```python
from build123d import *

# Parameters (mm, degrees)
CROQUIS2_R              = 10
SALIENTE_EXTRUIR1_DEPTH = 30
SALIENTE_EXTRUIR2_DEPTH = 2.5
CROQUIS4_W              = 3.81
CROQUIS4_H              = 5
CROQUIS5_W              = 70
CROQUIS5_H              = 20
SALIENTE_EXTRUIR3_DEPTH = 10
CORTAR_EXTRUIR1_DEPTH   = 20


with BuildPart() as part:
    # Croquis2 → Saliente-Extruir1 (new, symmetric)
    with BuildSketch(Plane(origin=(0, 0, 0), x_dir=(1, 0, 0), z_dir=(0, 1, 0))):
        with Locations(Location((0, 0, 0), (0, 0, 270))):
            Circle(CROQUIS2_R)
    extrude(amount=SALIENTE_EXTRUIR1_DEPTH, both=True)

    # Croquis3 → Saliente-Extruir2 (add, symmetric)
    with BuildSketch(Plane.XY):
        with BuildLine():
            Line((-1.082739864, -40.663757777), (-7.62, -30))
            Line((-7.62, -30), (7.62, -30))
            Line((7.62, -30), (1.082739864, -40.663757777))
            ThreePointArc((1.082739864, -40.663757777), (0, -41.27), (-1.082739864, -40.663757777))
        make_face()
    extrude(amount=SALIENTE_EXTRUIR2_DEPTH, both=True)

    # Croquis4 → Revoluci_n1 (revolve)
    with BuildSketch(Plane.XY, mode=Mode.PRIVATE) as revoluci_n1_sk:
        with Locations((11.905, -22.5)):
            Rectangle(CROQUIS4_W, CROQUIS4_H)
    revolve(revoluci_n1_sk.sketch.rotate(Axis((0, -30, 0), (0, -1, 0)), 90), axis=Axis((0, -30, 0), (0, -1, 0)))

    # Croquis5 → Saliente-Extruir3 (add)
    with BuildSketch(Plane(origin=(0, 30, 0), x_dir=(1, 0, 0), z_dir=(0, 1, 0))):
        Rectangle(CROQUIS5_W, CROQUIS5_H)
    extrude(amount=SALIENTE_EXTRUIR3_DEPTH)

    # Croquis6 → Cortar-Extruir1 (cut)
    with BuildSketch(Plane.XY.offset(10)):
        Polygon((35, 30), (15, 40), (35, 40), align=None)
    extrude(amount=-CORTAR_EXTRUIR1_DEPTH, mode=Mode.SUBTRACT)


solid = part.part
```
Could you check a few things on this model? Use its own coordinates, in mm. A direction names the side the tool comes from. Give positions to 0.01 mm unless a question says otherwise; leave off trailing zeros. Order: outer loops, then holes, each group sorted by start corner. A loop starts at its lowest first (then second) coordinate and runs counter-clockwise, first axis right, second up.
Q1. Suppose I cut it at C-C, the plane x = 20.5. Write out the boundary of the cut face in (y, z), and give its area (3 significant figures).
Q2. If I drill on line 1 along Y through (x, z) = (-10, 2.75); line 2 along Y through (x, z) = (-18.5, -6.5); line 3 along Z through (x, y) = (-26.5, 35), over which ranges is the centre line in solid material (lowest first)?
Q3. Suppose I cut it at B-B, the plane y = -2. Write out the boundary of the cut face in (x, z).
Q4. For faces 1 (the cylindrical face through (-9.76, 5.35, -2.17)), 2 (the flat face through (0, -34, -2.5)), 3 (the flat face through (-8, 35, -10)), 4 (the flat face through (-8, 35, 10)), which set-ups out of +Z, -Z, +X, -X, +Y, -Y let a thin tool reach every point of the face, with its end or its side?
Q5. Suppose I cut it at A-A, the plane z = 0. Write out the boundary of the cut face in (x, y).
Q6. Suppose I cut it at D-D, the plane z = 4. Write out the boundary of the cut face in (x, y), and give its area (3 significant figures).
Q7. We'd pull the mould along Y, two halves only. Please class faces 5 (the cylindrical face through (0.02, -41.27, 0.04)), 6 (the flat face through (-4.2, -20, 9.3)), 7 (the flat face through (25, 35, 0)), 8 (the cylindrical face through (-9.76, -27.46, -2.17)): +Y half, -Y half, draft (parallel to the pull), parting line (faces both ways), or undercut.
Q8. I'm going to push flat-ended pins straight in: P1, Ø2, axis at y = -13, z = 0.5, coming from the -X side; P2, Ø12, axis at y = -22.5, z = 2, coming from the +X side; P3, Ø8, axis at x = 9.5, y = -32, coming from the +Z side. Where does each tip first touch, or does it pass through?
Solution:
1. outline: (30, -10) - (37.25, -10) - (37.25, 10) - (30, 10) - close
1. area: 145 mm2
2. line 1: y = -25 to -20, 30 to 40
2. line 2: y = 30 to 40
2. line 3: z = -10 to 10
3. outline: circle Ø20 at (0, 0)
4. face 1: none
4. face 2: -Z, +X, -X, -Y
4. face 3: -Z, +X, -X, +Y
4. face 4: +Z, +X, -X, +Y
5. outline: (-35, 30) - (-10, 30) - (-10, -20) - (-13.81, -20) - (-13.81, -25) - (-10, -25) - (-10, -30) - (-7.62, -30) - (-1.08, -40.66) arc R1.27 ccw to (1.08, -40.66) - (7.62, -30) - (10, -30) - (10, -25) - (13.81, -25) - (13.81, -20) - (10, -20) - (10, 30) - (35, 30) - (15, 40) - (-35, 40) - close
6. outline: (-35, 30) - (-9.17, 30) - (-9.17, -20) - (-13.22, -20) - (-13.22, -25) - (-9.17, -25) - (-9.17, -30) - (9.17, -30) - (9.17, -25) - (13.22, -25) - (13.22, -20) - (9.17, -20) - (9.17, 30) - (35, 30) - (15, 40) - (-35, 40) - close
6. area: 1,740 mm2
7. face 5: -Y half
7. face 6: undercut
7. face 7: +Y half
7. face 8: draft
8. P1: stops at x = -10
8. P2: stops at x = 13.81
8. P3: stops at z = 7.97
